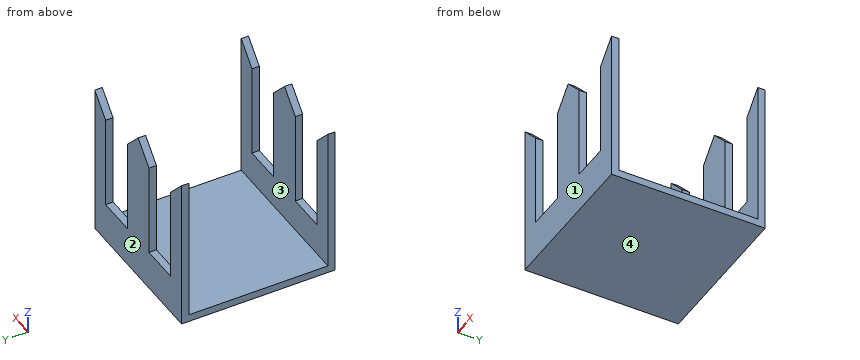
from build123d import *

# Parameters (mm, degrees)
F1_DEPTH = 76.2
F2_W     = 68.889363
F2_H     = 4.894324
F2_H_2   = 72.643043
F3_DEPTH = 88.9


with BuildPart() as f1:
    # F0 (on Front) → F1 (new body)
    with BuildSketch(Plane.XZ):
        Polygon((0, 76.288603), (0, 0), (76.19068, 0), (76.19068, 76.288603), (66.666845, 66.201665), (66.666845, 19.684223), (47.619175, 19.684223), (47.619175, 66.201665), (38.09534, 76.288603), (28.571505, 66.201665), (28.571505, 19.684223), (9.523835, 19.684223), (9.523835, 66.201665), align=None)
    extrude(amount=F1_DEPTH)

    # F2 (on face) → F3 (cut)
    with BuildSketch(Plane.YZ.offset(76.19068)):
        with Locations((-38.141334, 78.735765)):
            Rectangle(F2_W, F2_H)
        with Locations((-38.141334, 39.967081)):
            Rectangle(F2_W, F2_H_2)
    extrude(amount=-F3_DEPTH, mode=Mode.SUBTRACT)


solid = f1.part
Design review of the part built by this model. Coordinates are the model's own, in mm. Face numbers are marked on the shaded views. Give positions to 0.01 mm unless a question says otherwise; leave off trailing zeros. Loops run counter-clockwise (first coordinate to the right, second up) from the corner with the lowest first, then second, coordinate; pieces in that order, holes last. Notation, with made-up numbers: (72.25, 58) -> (115.25, 58) arc R23 cw to (115.25, 91) -> close; hole circle Ø11 at (1.5, 49). An arc over 180 degrees is marked (long way). One line per question, with ' | ' between items. Start each with the question number.
(1) Draft analysis for pull direction Y (two halves, no side actions). For the marked faces 1, 2, 3 and 4, state which applies: +Y half, -Y half, draft (parallel to the pull), parting line (faces both ways), or undercut.
(2) For line 1 (X direction, y = -73, z = 58.5); line 2 (Y direction, x = 40, z = 14); line 3 (Z direction, x = 48, y = -72), list the stretches that pass through material, from the lowest coordinate up.
(3) We need section D-D (y = -13). State the section outline as (x, z) points.
(4) We need section C-C (x = 64.5). State the section outline as (y, z) points, and give its area (3 significant figures).
(5) Insertion check: P1, Ø1.1, axis at x = 54, y = -1.5, coming from the +Z side. The pin has a flat end and moves straight along its axis. Give the tip position at first contact, or say it passes through.
(6) We need section A-A (z = 9). State the section outline as (x, y) points, and give its area (3 significant figures).
(7) We need section B-B (z = 31.5). State the section outline as (x, y) points.
The answers:
1) face 1: -Y half | face 2: +Y half | face 3: undercut | face 4: draft
2) line 1: x = 0 to 9.52, 28.57 to 47.62, 66.67 to 76.19 | line 2: y = -76.2 to -72.59, -3.7 to 0 | line 3: z = 0 to 3.65
3) outline: (0, 0) -> (76.19, 0) -> (76.19, 3.65) -> (0, 3.65) -> close
4) outline: (-76.2, 0) -> (0, 0) -> (0, 19.68) -> (-3.7, 19.68) -> (-3.7, 3.65) -> (-72.59, 3.65) -> (-72.59, 19.68) -> (-76.2, 19.68) -> close | area: 395 mm^2
5) P1: stops at z = 19.68
6) outline: (0, -76.2) -> (76.19, -76.2) -> (76.19, -72.59) -> (0, -72.59) -> close; (0, -3.7) -> (76.19, -3.7) -> (76.19, 0) -> (0, 0) -> close | area: 557 mm^2
7) outline: (0, -76.2) -> (9.52, -76.2) -> (9.52, -72.59) -> (0, -72.59) -> close; (0, -3.7) -> (9.52, -3.7) -> (9.52, 0) -> (0, 0) -> close; (28.57, -76.2) -> (47.62, -76.2) -> (47.62, -72.59) -> (28.57, -72.59) -> close; (28.57, -3.7) -> (47.62, -3.7) -> (47.62, 0) -> (28.57, 0) -> close; (66.67, -76.2) -> (76.19, -76.2) -> (76.19, -72.59) -> (66.67, -72.59) -> close; (66.67, -3.7) -> (76.19, -3.7) -> (76.19, 0) -> (66.67, 0) -> close
